```python
from build123d import *

# Parameters (mm, degrees)
BOSS_EXTRUDE1_DEPTH     = 2.54
CUT_EXTRUDE1_DEPTH      = 112.420336115
CUT_EXTRUDE1_DEPTH_BACK = 112.420336115
SKETCH11_W              = 3.81
SKETCH11_H              = 11.43
SKETCH11_W_2            = 8.382
SKETCH11_H_2            = 8.382
CUT_EXTRUDE2_DEPTH      = 112.420336115
CUT_EXTRUDE2_DEPTH_BACK = 112.420336115
SKETCH12_R              = 1.27
CUT_EXTRUDE3_DEPTH      = 112.420336115
CUT_EXTRUDE3_DEPTH_BACK = 112.420336115
SKETCH13_R              = 1.27
CUT_EXTRUDE4_DEPTH      = 112.420336115
CUT_EXTRUDE4_DEPTH_BACK = 112.420336115
SKETCH14_W              = 3.556
SKETCH14_H              = 13.97


with BuildPart() as part:
    # Sketch10 → Boss-Extrude1 (new body)
    with BuildSketch(Plane.XY):
        with BuildLine():
            Line((53.34, 1.27), (53.34, -92.71))
            ThreePointArc((53.34, -92.71), (51.852102448, -96.302102448), (48.26, -97.79))
            Line((48.26, -97.79), (16.846989059, -97.79))
            ThreePointArc((16.846989059, -97.79), (15.638688158, -97.644208035), (14.499741809, -97.215200367))
            Line((14.499741809, -97.215200367), (-16.7505185, -80.933552139))
            ThreePointArc((-16.7505185, -80.933552139), (-18.059258376, -79.955412607), (-18.989802686, -78.61241436))
            Line((-18.989802686, -78.61241436), (-28.309569459, -59.040904135))
            ThreePointArc((-28.309569459, -59.040904135), (-28.795802898, -57.127870198), (-28.51617555, -55.173917704))
            Line((-28.51617555, -55.173917704), (-8.107195629, 2.952923842))
            ThreePointArc((-8.107195629, 2.952923842), (-6.251501454, 5.414614163), (-3.314058103, 6.35))
            Line((-3.314058103, 6.35), (48.26, 6.35))
            ThreePointArc((48.26, 6.35), (51.852102448, 4.862102448), (53.34, 1.27))
        make_face()
    extrude(amount=BOSS_EXTRUDE1_DEPTH)

    # Sketch11 → Cut-Extrude1 (cut, two sides: drawn at the far end of the back side and taken through both)
    with BuildSketch(Plane.XY.offset(2.54).offset(-CUT_EXTRUDE1_DEPTH_BACK)):
        with Locations((31.65602, -79.121)):
            Rectangle(SKETCH11_W, SKETCH11_H)
        with Locations((23.78202, -79.121)):
            Rectangle(SKETCH11_W, SKETCH11_H)
        with Locations((3.878385852, -55.88)):
            Rectangle(SKETCH11_W_2, SKETCH11_H_2)
        with Locations((-5.011614148, -46.99)):
            Rectangle(SKETCH11_W_2, SKETCH11_H_2)
        with Locations((3.878385852, -38.1)):
            Rectangle(SKETCH11_W_2, SKETCH11_H_2)
        with Locations((12.768385852, -46.99)):
            Rectangle(SKETCH11_W_2, SKETCH11_H_2)
        with Locations((-9.017, -64.897)):
            Rectangle(SKETCH11_W_2, SKETCH11_H_2)
        with Locations((3.175, -70.485)):
            Rectangle(SKETCH11_W_2, SKETCH11_H_2)
        with Locations((15.367, -76.073)):
            Rectangle(SKETCH11_W_2, SKETCH11_H_2)
    extrude(amount=CUT_EXTRUDE1_DEPTH + CUT_EXTRUDE1_DEPTH_BACK, mode=Mode.SUBTRACT)

    # Sketch12 → Cut-Extrude2 (cut, two sides: drawn at the far end of the back side and taken through both)
    with BuildSketch(Plane(origin=(0, 0, 0), x_dir=(-1, 0, 0), z_dir=(0, 0, -1)).offset(-CUT_EXTRUDE2_DEPTH_BACK)):
        with Locations((18.034, -57.15)):
            Circle(SKETCH12_R)
        with Locations((-43.942, -85.852)):
            Circle(SKETCH12_R)
    extrude(amount=CUT_EXTRUDE2_DEPTH + CUT_EXTRUDE2_DEPTH_BACK, mode=Mode.SUBTRACT)

    # Sketch13 → Cut-Extrude3 (cut, two sides: drawn at the far end of the back side and taken through both)
    with BuildSketch(Plane(origin=(0, 0, 0), x_dir=(-1, 0, 0), z_dir=(0, 0, -1)).offset(-CUT_EXTRUDE3_DEPTH_BACK)):
        with Locations((25.012261453, -59.761967182)):
            Circle(SKETCH13_R)
        with Locations((-48.0822, 2.286)):
            Circle(SKETCH13_R)
        with Locations((3.718687848, 1.651)):
            Circle(SKETCH13_R)
    extrude(amount=CUT_EXTRUDE3_DEPTH + CUT_EXTRUDE3_DEPTH_BACK, mode=Mode.SUBTRACT)

    # Sketch14 → Cut-Extrude4 (cut, two sides: drawn at the far end of the back side and taken through both)
    with BuildSketch(Plane(origin=(0, 0, 0), x_dir=(-1, 0, 0), z_dir=(0, 0, -1)).offset(-CUT_EXTRUDE4_DEPTH_BACK)):
        with Locations((-35.010498686, -19.798068862)):
            Rectangle(SKETCH14_W, SKETCH14_H)
    extrude(amount=CUT_EXTRUDE4_DEPTH + CUT_EXTRUDE4_DEPTH_BACK, mode=Mode.SUBTRACT)


solid = part.part
```
Verification items for the finished model (mm, model axes). A direction names the side the tool comes from. Round coordinates to 2 decimals unless told otherwise and drop trailing zeros. Write each loop counter-clockwise with the first axis right and the second up, starting at its lowest first coordinate (ties: lowest second). Pieces come first, ordered by that corner, then holes. Notation, with made-up numbers: (-38.75, -17) - (2.25, -17) arc R18 cw to (2.25, -8) - close; hole circle Ø4 at (-7.5, 61.5). An arc over 180 degrees is marked (long way). Answer as a JSON object with one key per item and string values. Group by question number.
Q1. Section check A-A, the plane y = -21.5. Enter the section's corners in (x, z).
Q2. Go/stop test with flat-tipped pins: pin 1 Ø3.5 at (x, y) = (43.942, -85.852) entering from +Z; pin 2 Ø1.3 at (y, z) = (-56, 0.5) entering from -X; pin 3 Ø1 at (y, z) = (-51.5, 1) entering from -X. Record where each tip stops, or that it passes through.
Q3. Tool access check on faces 1 (the flat face through (3, -74.676, 1)), 2 (the flat face through (22, -45, 0)). Record the directions out of +Z, -Z, +X, -X, +Y, -Y that give a thin tool (end or side, any length) a straight path to the whole face; none if there is none.
Q4. Thickness scan on line 1 (X direction, y = -57.15, z = 2); line 2 (Y direction, x = 1, z = 1); line 3 (Y direction, x = -5.5, z = 0.35). Record the ranges inside material, lowest first.
Q5. Section check D-D, the plane z = 1.3. Give the number of separate pieces and of enclosed holes in the cut face, plus the area to 3 significant figures.
Q6. Section check B-B, the plane y = -57.15. Enter the section's corners in (x, z), plus the area to 3 significant figures.
Q7. Mould release check, pull along X, two halves, no side actions. Record for faces 3 (the flat face through (33, -97.79, 1)), 4 (the flat face through (32, -73.406, 1)), 5 (the cylindrical face through (-6.287, 5.389, 1.252)): released by +X, released by -X, zero draft, split by the parting line, or undercut.
Q8. Section check C-C, the plane y = -38.5. Enter the section's corners in (x, z), plus the area to 3 significant figures.
Found:
{
 "1": {"outline": "(-16.69, 0) - (33.23, 0) - (33.23, 2.54) - (-16.69, 2.54) - close; (36.79, 0) - (53.34, 0) - (53.34, 2.54) - (36.79, 2.54) - close"},
 "2": {"pin 1": "stops at z = 2.54", "pin 2": "stops at x = -28.8", "pin 3": "stops at x = -27.4"},
 "3": {"face 1": "+Z, -Z", "face 2": "-Z, +X, -X, +Y, -Y"},
 "4": {"line 1": "x = -28.79 to -19.3, -16.76 to -0.31, 8.07 to 53.34", "line 2": "y = -90.18 to -74.68, -66.29 to -60.07, -51.69 to -42.29, -33.91 to 6.35", "line 3": "y = -86.8 to -69.09, -60.71 to -51.18, -42.8 to 5.86"},
 "5": {"separate pieces": "1", "enclosed holes": "15", "area": "6,600 mm^2"},
 "6": {"outline": "(-28.79, 0) - (-19.3, 0) - (-19.3, 2.54) - (-28.79, 2.54) - close; (-16.76, 0) - (-0.31, 0) - (-0.31, 2.54) - (-16.76, 2.54) - close; (8.07, 0) - (53.34, 0) - (53.34, 2.54) - (8.07, 2.54) - close", "area": "181 mm^2"},
 "7": {"face 3": "zero draft", "face 4": "undercut", "face 5": "released by -X"},
 "8": {"outline": "(-22.66, 0) - (-0.31, 0) - (-0.31, 2.54) - (-22.66, 2.54) - close; (8.07, 0) - (53.34, 0) - (53.34, 2.54) - (8.07, 2.54) - close", "area": "172 mm^2"}
}
